Autodesk Inventor part; units mm, degrees
ref_plane "YZ Plane" through (0, 0, 0) normal (1, 0, 0) x (0, 1, 0)
ref_plane "XZ Plane" through (0, 0, 0) normal (0, 1, 0) x (-1, 0, 0)
ref_plane "XY Plane" through (0, 0, 0) normal (0, 0, 1) x (1, 0, 0)
sketch "Sketch1" plane through (0, 0, 0) normal (0, 1, 0) x (-1, 0, 0)
  line L0 (37.6, 60.35) -> (-37.6, 60.35)
  line L1 (-37.6, 60.35) -> (-37.6, -60.35)
  line L2 (-37.6, -60.35) -> (37.6, -60.35)
  line L3 (37.6, -60.35) -> (37.6, 60.35)
  line L4 (37.6, 60.35) -> (-37.6, -60.35) construction
  line L5 (-37.6, 60.35) -> (37.6, -60.35) construction
  line L6 (39.6, 62.35) -> (-39.6, 62.35)
  line L7 (-39.6, 62.35) -> (-39.6, -62.35)
  line L8 (-39.6, -62.35) -> (39.6, -62.35)
  line L9 (39.6, -62.35) -> (39.6, 62.35)
  point P0 (0, 0)
  dimension "d0" = 120.7
  dimension "d1" = 75.2
  dimension "d2" = 2
  dimension "d3" = 2
  dimension "d4" = 2
  dimension "d5" = 2
extrude "Extrusion1" add sketch "Sketch1" along normal blind 35
sketch "Sketch4" plane through (0, 0, 0) normal (0, -1, 0) x (1, 0, 0)
  line L0 (-39.6, 62.35) -> (39.6, 62.35)
  line L1 (39.6, 62.35) -> (-39.6, 62.35)
  line L2 (-39.6, 62.35) -> (-39.6, -62.35)
  line L3 (-39.6, -62.35) -> (39.6, -62.35)
  line L4 (39.6, -62.35) -> (39.6, 62.35)
  circle A0 centre (0, -32.35) radius 5.1
  line L5 (-37.6, 60.35) -> (-37.6, -60.35)
  point P0 (0, 0)
  point P1 (-39.6, 62.35)
  dimension "d13" = 10.2
  dimension "d14" = 37.6
  dimension "d15" = 30
extrude "Extrusion3" add sketch "Sketch4" along normal blind 2
Input: part model. Units: mm. Frame: model coordinates. A direction names the side the tool comes from. Give positions to 0.01 mm unless a question says otherwise; leave off trailing zeros. Write each loop counter-clockwise with the first axis right and the second up, starting at its lowest first coordinate (ties: lowest second). Pieces come first, ordered by that corner, then holes. Notation, with made-up numbers: (7, 13.25) - (41, 13.25) arc R19 cw to (41, 48.25) - close; hole circle Ø5 at (-36.75, 75). An arc over 180 degrees is marked (long way). Write item = value, one per line. Start each with the question number.
1. Section query D-D, the plane z = 24. Output: boundary loops of the cut face in (x, y), then the cut area to 3 significant figures.
2. Access query for faces 5 (the flat face through (39.6, 16, 1)), 6 (the flat face through (37.6, 17, 1)). Directions: +Z, -Z, +X, -X, +Y, -Y. A direction counts if a zero-diameter tool reaches every point of the face in a straight line with its end or side. Return the directions, or none.
3. Mould query, pull axis X, two halves, no side actions, for faces 1 (the flat face through (-39.6, 16, -1)), 2 (the flat face through (1, 17, -60.35)), 3 (the flat face through (-37.6, 17, -1)), 4 (the flat face through (-38, 35, 0)). Classes: released by +X, released by -X, zero draft, split by the parting line, or undercut.
4. Section query A-A, the plane x = 0. Output: boundary loops of the cut face in (y, z).
5. Section query B-B, the plane z = -32.35. Output: boundary loops of the cut face in (x, y), then the cut area to 3 significant figures.
6. Section query C-C, the plane y = 12.5. Output: boundary loops of the cut face in (x, z), then the cut area to 3 significant figures.
7. First-contact query: pin 1 Ø10 at (x, z) = (21.5, 1) entering from +Y. Flat tip, straight axial feed; report the tip coordinate or a pass-through.
8. Ray query, L1, parallel to Z at x = -32, y = 31.5; L2, parallel to X at y = 26, z = -6; L3, parallel to Z at x = 0, y = -1. Return the intervals inside material, ascending.
Check sheet entries:
q1.outline = (-39.6, -2) - (39.6, -2) - (39.6, 35) - (37.6, 35) - (37.6, 0) - (-37.6, 0) - (-37.6, 35) - (-39.6, 35) - close
q1.area = 298 mm2
q2.face_5 = +Z, -Z, +X, +Y, -Y
q2.face_6 = +Y
q3.face_1 = released by -X
q3.face_2 = undercut
q3.face_3 = undercut
q3.face_4 = zero draft
q4.outline = (-2, -62.35) - (35, -62.35) - (35, -60.35) - (0, -60.35) - (0, -37.45) - (-2, -37.45) - close; (-2, -27.25) - (0, -27.25) - (0, 60.35) - (35, 60.35) - (35, 62.35) - (-2, 62.35) - close
q5.outline = (-39.6, -2) - (-5.1, -2) - (-5.1, 0) - (-37.6, 0) - (-37.6, 35) - (-39.6, 35) - close; (5.1, -2) - (39.6, -2) - (39.6, 35) - (37.6, 35) - (37.6, 0) - (5.1, 0) - close
q5.area = 278 mm2
q6.outline = (-39.6, -62.35) - (39.6, -62.35) - (39.6, 62.35) - (-39.6, 62.35) - close; hole (-37.6, -60.35) - (37.6, -60.35) - (37.6, 60.35) - (-37.6, 60.35) - close
q6.area = 800 mm2
q7.pin_1 = 0
q8.L1 = -62.35 to -60.35, 60.35 to 62.35
q8.L2 = -39.6 to -37.6, 37.6 to 39.6
q8.L3 = -62.35 to -37.45, -27.25 to 62.35
